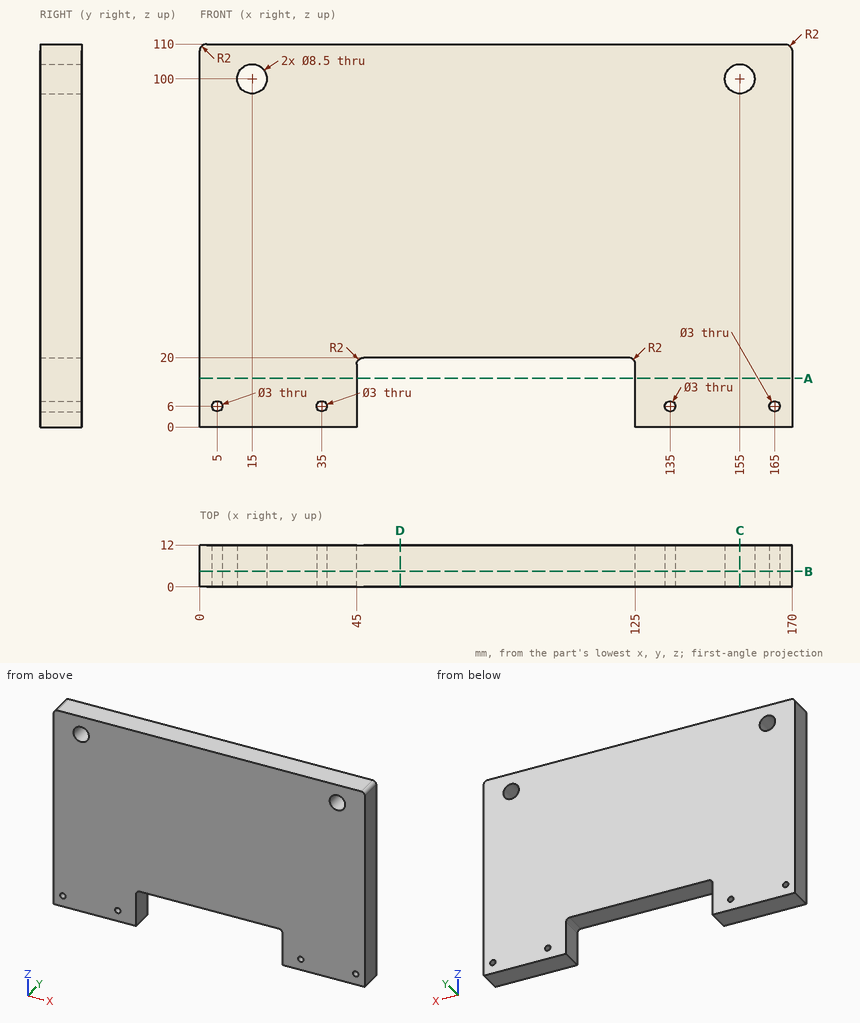
Design review of the part shown in the three views and the two pictorial views. Dimensions are in mm from the part's minimum x, y and z. Round coordinates to 2 decimals unless told otherwise and drop trailing zeros. Loops run counter-clockwise (first coordinate to the right, second up) from the corner with the lowest first, then second, coordinate; pieces in that order, holes last. Notation, with made-up numbers: M 34.25,-34 L 92.25,-34 A20 cw 92.25,-9 Z; hole C -14.75,-5 d6. An arc over 180 degrees is marked long. Put each result on its own line as item: value.
Q1. To check wall thickness, follow L1, parallel to X at y = 3, z = 6; L2, parallel to X at y = 4, z = 100; L3, parallel to X at y = 5.5, z = 13. State the ranges of each line that lie inside material, in increasing order.
Result set:
L1: x = 0 to 3.5, 6.5 to 33.5, 36.5 to 45, 125 to 133.5, 136.5 to 163.5, 166.5 to 170
L2: x = 0 to 10.75, 19.25 to 150.75, 159.25 to 170
L3: x = 0 to 45, 125 to 170
Q2. For pin 1 (1.8 mm diameter, centred on x = 165, z = 6, fed in from -Y), flat-tipped, find the tip position at first contact; note if it passes through.
Result set:
pin 1: passes through
Q3. Consider section D-D, the plane x = 57.5. Give the boundary of the cut face in (y, z).
Result set:
outline: M 0,20 L 12,20 L 12,110 L 0,110 Z
Q4. Consider section B-B, the plane y = 4.5. Give the boundary of the cut face in (x, z).
Result set:
outline: M 0,0 L 45,0 L 45,18 A2 cw 47,20 L 123,20 A2 cw 125,18 L 125,0 L 170,0 L 170,108 A2 ccw 168,110 L 2,110 A2 ccw 0,108 Z; hole C 5,6 d3; hole C 15,100 d8.5; hole C 35,6 d3; hole C 135,6 d3; hole C 155,100 d8.5; hole C 165,6 d3
Q5. Consider section A-A, the plane z = 14. Give the boundary of the cut face in (x, y), then the cut area to 3 significant figures.
Result set:
outline: M 0,0 L 45,0 L 45,12 L 0,12 Z; M 125,0 L 170,0 L 170,12 L 125,12 Z
area: 1,080 mm²
Q6. Consider section C-C, the plane x = 155. Give the boundary of the cut face in (y, z).
Result set:
outline: M 0,0 L 12,0 L 12,95.75 L 0,95.75 Z; M 0,104.25 L 12,104.25 L 12,110 L 0,110 Z
